from build123d import *

# Parameters (mm, degrees)
F1_DEPTH = 78.232
F2_DEPTH = 62.484
F3_DEPTH = 62.484


with BuildPart() as f1:
    # F0 (on Top) → F1 (new body)
    with BuildSketch(Plane.XY):
        Polygon((-36.178753, 33.396009), (-47.011169, -14.633714), (-10.832416, -48.029724), (36.178753, -33.396009), (47.011169, 14.633714), (10.832416, 48.029724), align=None)
    extrude(amount=F1_DEPTH)

    # F0 (on Top) → F2 (join)
    with BuildSketch(Plane.XY):
        Polygon((-10.832416, -48.029724), (-47.011169, -14.633714), (-35.825498, -49.588244), align=None)
    extrude(amount=F2_DEPTH)

    # F0 (on Top) → F3 (join)
    with BuildSketch(Plane.XY):
        Polygon((47.011169, 14.633714), (36.178753, -33.396009), (60.519096, -11.588277), align=None)
    extrude(amount=F3_DEPTH)


solid = f1.part
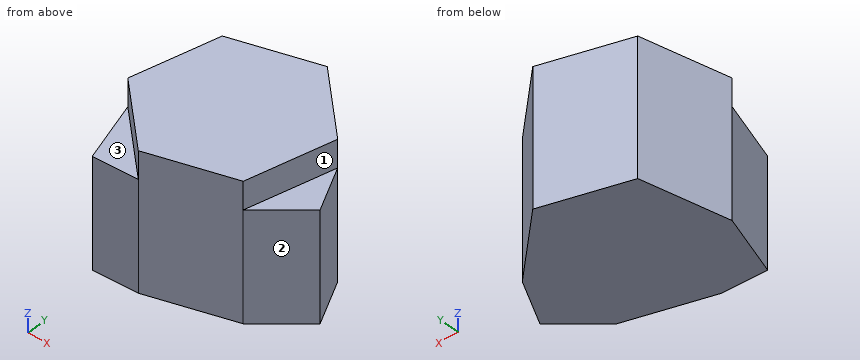
Build history of the part. All positions in model axes, mm. Face numbers are marked on the shaded views. A direction names the side the tool comes from. Give positions to 0.01 mm unless a question says otherwise; leave off trailing zeros. Loops run counter-clockwise (first coordinate to the right, second up) from the corner with the lowest first, then second, coordinate; pieces in that order, holes last. Notation, with made-up numbers: (21.25, 60.5) - (53.25, 60.5) arc R20 ccw to (53.25, 97.5) - close; hole circle Ø2 at (-38, -10.75). An arc over 180 degrees is marked (long way). Write item = value, one per line. Start each with the question number.
1) Probe probe 1 along X at (y, z) = (-13.5, 59.5); probe 2 along Y at (x, z) = (29, 75.5); probe 3 along Y at (x, z) = (23.5, 9.5). List the from-to ranges inside material, lowest first. Write a range as from..to.
2) Drop flat-ended pins along their axis: pin 1 Ø2 at (y, z) = (35.5, 34) entering from +X; pin 2 Ø2 at (y, z) = (-26.5, 46.5) entering from +X; pin 3 Ø12 at (y, z) = (7, 8.5) entering from -X. Give the stop position or say it passes through.
3) Band-saw the part on C-C on x = -24. Give the cut face in (y, z).
4) Tool access for the marked faces 1, 2 and 3: list every direction of +Z, -Z, +X, -X, +Y, -Y with a clear straight run to the whole face (end or side of a thin tool).
5) Band-saw the part on D-D on x = -38. Give the cut face in (y, z), plus the area to 3 significant figures.
6) Band-saw the part on A-A on z = 39.5. Give the cut face in (x, y).
7) Band-saw the part on B-B on y = -30.5. Give the cut face in (x, z).
Final values:
q1.probe_1 = -46.76..58.39
q1.probe_2 = -35.63..31.26
q1.probe_3 = -37.34..36.34
q2.pin_1 = 25.49
q2.pin_2 = 44.99
q2.pin_3 = -43.49
q3.outline = (-48.85, 0) - (37.19, 0) - (37.19, 78.23) - (-35.87, 78.23) - (-35.87, 62.48) - (-48.85, 62.48) - close
q4.face_1 = +Z, +X, -Y
q4.face_2 = +Z, -Z, +X, -Y
q4.face_3 = +Z, -X, -Y
q5.outline = (-42.79, 0) - (25.32, 0) - (25.32, 78.23) - (-22.95, 78.23) - (-22.95, 62.48) - (-42.79, 62.48) - close
q5.area = 5,020 mm²
q6.outline = (-47.01, -14.63) - (-35.83, -49.59) - (-10.83, -48.03) - (36.18, -33.4) - (60.52, -11.59) - (47.01, 14.63) - (10.83, 48.03) - (-36.18, 33.4) - close
q7.outline = (-41.93, 0) - (39.41, 0) - (39.41, 62.48) - (36.83, 62.48) - (36.83, 78.23) - (-29.82, 78.23) - (-29.82, 62.48) - (-41.93, 62.48) - close
